Can you work these out from the model? Positions are in its coordinate system, mm. Face numbers are marked on the shaded views. A direction names the side the tool comes from. Give positions to 0.01 mm unless a question says otherwise; leave off trailing zeros. Write each loop counter-clockwise with the first axis right and the second up, starting at its lowest first coordinate (ties: lowest second). Pieces come first, ordered by that corner, then holes.
1. I'm going to push a flat-ended pin straight in: pin 1 (2 mm diameter, centred on x = 1420.5, y = 1171, fed in from +Z). Where does the tip first touch, or does it pass through?
2. Thinking about a two-plate mould opening in Y: for the marked faces 1, 2, 3 and 4, which applies, pulls with the +Y half, pulls with the -Y half, needs draft (parallel to the pull), parting line crosses it, or undercut?
3. Suppose I cut it at D-D (y = 1562.1). Please give me the cut outline in (x, z), and give its area (3 significant figures).
4. If I drill on probe 1 along Y at (x, z) = (1365.25, 218); probe 2 along X at (y, z) = (254, 343); probe 3 along X at (y, z) = (1879.5, 386.5), over which ranges is the centre line in solid material (lowest first)?
5. Suppose I cut it at C-C (z = 587.5). Please give me the cut outline in (x, y).
6. Suppose I cut it at B-B (x = 1365.25). Please give me the cut outline in (y, z), and give its area (3 significant figures).
7. On a 3-axis mill with a long thin cutter (end or side, diameter ignored), from which of +Z, -Z, +X, -X, +Y, -Y can I reach the whole of each face in a straight line? I mean the marked faces 5, 6 and 7. Say none if no direction works.
8. Suppose I cut it at A-A (y = 1905). Please give me the cut outline in (x, z), and give its area (3 significant figures).
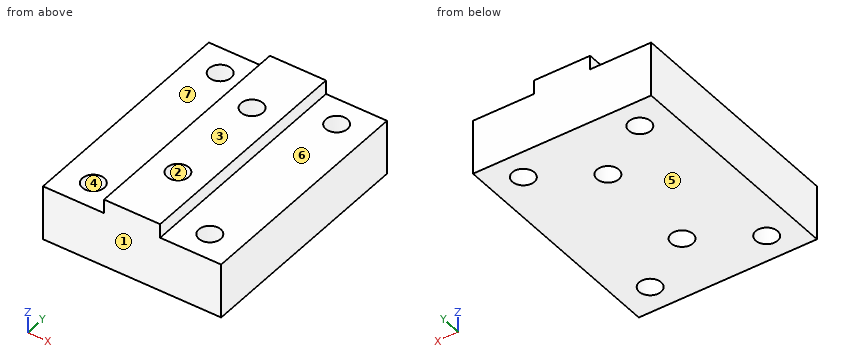
```python
from build123d import *

# Parameters (mm, degrees)
SKETCH1_W           = 1651
SKETCH1_H           = 2159
SKETCH1_R           = 101.6
BOSS_EXTRUDE1_DEPTH = 508
BOSS_EXTRUDE2_START = 130
SKETCH2_W           = 520
SKETCH2_H           = 2159
SKETCH2_R           = 101.6
BOSS_EXTRUDE2_DEPTH = 130


with BuildPart() as part:
    # Sketch1 → Boss-Extrude1 (new body)
    with BuildSketch(Plane.XY.offset(508)):
        with Locations((825.5, 1079.5)):
            Rectangle(SKETCH1_W, SKETCH1_H)
        with Locations(Location((285.75, 254, 0), (0, 0, 180))):
            Circle(SKETCH1_R, mode=Mode.SUBTRACT)
        with Locations(Location((1365.25, 1905, 0), (0, 0, 180))):
            Circle(SKETCH1_R, mode=Mode.SUBTRACT)
        with Locations(Location((825.5, 1562.1, 0), (0, 0, 180))):
            Circle(SKETCH1_R, mode=Mode.SUBTRACT)
        with Locations(Location((285.75, 1905, 0), (0, 0, 180))):
            Circle(SKETCH1_R, mode=Mode.SUBTRACT)
        with Locations(Location((1365.25, 254, 0), (0, 0, 180))):
            Circle(SKETCH1_R, mode=Mode.SUBTRACT)
        with Locations(Location((825.5, 596.9, 0), (0, 0, 180))):
            Circle(SKETCH1_R, mode=Mode.SUBTRACT)
    extrude(amount=-BOSS_EXTRUDE1_DEPTH)

    # Sketch2 → Boss-Extrude2 (add)
    with BuildSketch(Plane.XY.offset(508).offset(BOSS_EXTRUDE2_START)):
        with Locations((825.5, 1079.5)):
            Rectangle(SKETCH2_W, SKETCH2_H)
        with Locations((825.5, 596.9)):
            Circle(SKETCH2_R, mode=Mode.SUBTRACT)
        with Locations((825.5, 1562.1)):
            Circle(SKETCH2_R, mode=Mode.SUBTRACT)
    extrude(amount=-BOSS_EXTRUDE2_DEPTH)


solid = part.part
```
Checks:
1. pin 1: stops at z = 508
2. face 1: pulls with the -Y half
2. face 2: undercut
2. face 3: needs draft
2. face 4: undercut
3. outline: (0, 0) - (723.9, 0) - (723.9, 638) - (565.5, 638) - (565.5, 508) - (0, 508) - close; (927.1, 0) - (1651, 0) - (1651, 508) - (1085.5, 508) - (1085.5, 638) - (927.1, 638) - close
3. area: 777,000 mm2
4. probe 1: y = 0 to 152.4, 355.6 to 1803.4, 2006.6 to 2159
4. probe 2: x = 0 to 184.15, 387.35 to 1263.65, 1466.85 to 1651
4. probe 3: x = 0 to 187.4, 384.1 to 1266.9, 1463.6 to 1651
5. outline: (565.5, 0) - (1085.5, 0) - (1085.5, 2159) - (565.5, 2159) - close; hole circle Ø203.2 at (825.5, 596.9); hole circle Ø203.2 at (825.5, 1562.1)
6. outline: (0, 0) - (152.4, 0) - (152.4, 508) - (0, 508) - close; (355.6, 0) - (1803.4, 0) - (1803.4, 508) - (355.6, 508) - close; (2006.6, 0) - (2159, 0) - (2159, 508) - (2006.6, 508) - close
6. area: 890,000 mm2
7. face 5: -Z, +X, -X, +Y, -Y
7. face 6: +Z, +X, +Y, -Y
7. face 7: +Z, -X, +Y, -Y
8. outline: (0, 0) - (184.15, 0) - (184.15, 508) - (0, 508) - close; (387.35, 0) - (1263.65, 0) - (1263.65, 508) - (1085.5, 508) - (1085.5, 638) - (565.5, 638) - (565.5, 508) - (387.35, 508) - close; (1466.85, 0) - (1651, 0) - (1651, 508) - (1466.85, 508) - close
8. area: 700,000 mm2
